For this review, take the finished solid that the model builds, in its own axes (mm). Round coordinates to 2 decimals unless told otherwise and drop trailing zeros. Order: outer loops, then holes, each group sorted by start corner. A loop starts at its lowest first (then second) coordinate and runs counter-clockwise, first axis right, second up. Notation, with made-up numbers: (-13.75, -0.75) - (37.25, -0.75) arc R21 cw to (37.25, 25.25) - close; hole circle Ø2 at (31.25, 65). An arc over 180 degrees is marked (long way). One line per question, with ' | ' between items.
```python
from build123d import *

# Parameters (mm, degrees)
F0_R     = 0.6223
F1_DEPTH = 228.6


with BuildPart() as f1:
    # F0 (on Right) → F1 (new body)
    with BuildSketch(Plane.YZ):
        Circle(F0_R)
    extrude(amount=-F1_DEPTH)


with BuildPart() as f2_1:
    # F2: copy of F1
    add(f1.part)


with BuildPart() as f3_1:
    # F3: copy of F1
    add(f1.part)


solid = f1.part
```
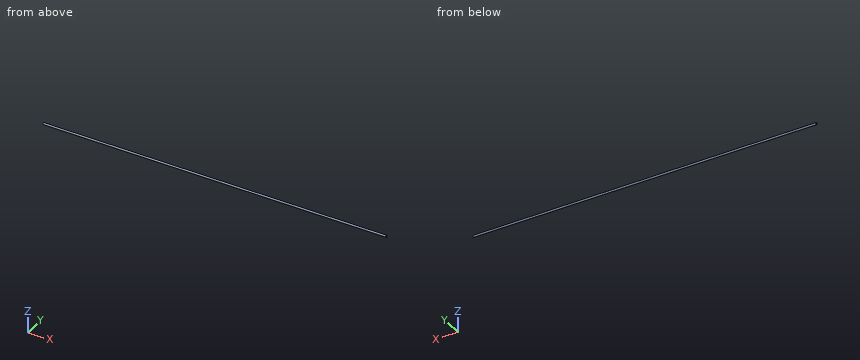
(1) For probe 1 along Y at (x, z) = (-173, -0.2); probe 2 along Y at (x, z) = (-125, 0.55), list the stretches that pass through material, from the lowest coordinate up. Write a range as [from, to].
Output values:
probe 1: [-0.59, 0.59] | probe 2: [-0.29, 0.29]
(2) We need section A-A on y = 0.3. State the section outline as (x, z) points.
Output values:
outline: (-228.6, -0.55) - (0, -0.55) - (0, 0.55) - (-228.6, 0.55) - close
(3) We need section B-B on x = -161.5. State the section outline as (y, z) points.
Output values:
outline: circle Ø1.24 at (0, 0)
